Verification items for the finished model (mm, model axes). A direction names the side the tool comes from. Round coordinates to 2 decimals unless told otherwise and drop trailing zeros. Write each loop counter-clockwise with the first axis right and the second up, starting at its lowest first coordinate (ties: lowest second). Pieces come first, ordered by that corner, then holes. Notation, with made-up numbers: M 65,-28.75 L 101,-28.75 A18 cw 101,-8.75 Z; hole C -15,28 d4. An arc over 180 degrees is marked long. Answer in a Markdown table with one row per item. Add a question column.
1. Go/stop test with flat-tipped pins: pin 1 Ø2 at (y, z) = (4, 0) entering from +X; pin 2 Ø1.2 at (y, z) = (-3.5, 0.5) entering from -X; pin 3 Ø4 at (x, y) = (-127, 0) entering from +Z; pin 4 Ø2 at (x, z) = (93, 1) entering from -Y. Record where each tip stops, or that it passes through.
2. Draft check along X on faces 1 (the flat face through (2, 0, 2)), 2 (the cylindrical face through (135, 0, 0)), 3 (the cylindrical face through (-110.3, 9.57, 0.03)). Enter one of: pulls with the +X half, pulls with the -X half, needs draft (parallel to the pull), parting line crosses it, or undercut.
3. Sectioned sample at B-B on z = -0.5. Count the separate pieces of the cut face and the enclosed holes in it, plus the area to 3 significant figures.
4. Material ranges on probe 1 along Y at (x, z) = (28.5, 0.2); probe 2 along X at (y, z) = (-12, -1.2); probe 3 along Y at (x, z) = (110.5, -0.1), recorded low to high.
5. Set-up check for faces 4 (the cylindrical face through (-135, 0, 0)), 5 (the cylindrical face through (101, -9, 0)): record each of +Z, -Z, +X, -X, +Y, -Y from which the full face is reachable in a straight line by a thin tool's end or side.
6. Sectioned sample at A-A on x = -127. Record the cut outline in (y, z), plus the area to 3 significant figures.
```python
from build123d import *

# Parameters (mm, degrees)
EXTRUDE_1_DEPTH     = 2
SKETCH_11_W         = 4.2
SKETCH_11_H         = 15
SKETCH_11_W_2       = 46.8
SKETCH_11_H_2       = 22
SKETCH_11_W_3       = 5
SKETCH_11_R         = 3.5
SKETCH_11_R_2       = 1.5
CUT_EXTRUDE_1_DEPTH = 10
SKETCH_12_W         = 45
SKETCH_12_H         = 22
EXTRUDE_2_DEPTH     = 4
SKETCH_13_W         = 4.1
SKETCH_13_H         = 15
CUT_EXTRUDE_2_DEPTH = 136.889661123
FILLET_1_R          = 5


with BuildPart() as part:
    # Эскиз1 → Бобышка-Вытянуть1 (new, symmetric)
    with BuildSketch(Plane.XY):
        with BuildLine():
            Line((-120, 15), (120, 15))
            ThreePointArc((120, 15), (135, 0), (120, -15))
            Line((120, -15), (-120, -15))
            ThreePointArc((-120, -15), (-135, 0), (-120, 15))
        make_face()
    extrude(amount=EXTRUDE_1_DEPTH, both=True)

    # Эскиз11 → Вырез-Вытянуть1 (cut)
    with BuildSketch(Plane(origin=(0, 0, -2), x_dir=(-1, 0, 0), z_dir=(0, 0, -1))):
        with Locations((-117.9, 7.5)):
            Rectangle(SKETCH_11_W, SKETCH_11_H)
        with Locations((-88.4, 0)):
            Rectangle(SKETCH_11_W_2, SKETCH_11_H_2)
        with Locations((-57.5, 0)):
            Rectangle(SKETCH_11_W_3, SKETCH_11_H_2)
        with Locations((-47.5, 0)):
            Rectangle(SKETCH_11_W_3, SKETCH_11_H_2)
        with Locations((-37.5, 0)):
            Rectangle(SKETCH_11_W_3, SKETCH_11_H_2)
        with Locations((-27.5, 0)):
            Rectangle(SKETCH_11_W_3, SKETCH_11_H_2)
        with Locations((-17.5, 0)):
            Rectangle(SKETCH_11_W_3, SKETCH_11_H_2)
        with Locations((-7.5, 0)):
            Rectangle(SKETCH_11_W_3, SKETCH_11_H_2)
        with Locations((7.5, 0)):
            Rectangle(SKETCH_11_W_3, SKETCH_11_H_2)
        with Locations((17.5, 0)):
            Rectangle(SKETCH_11_W_3, SKETCH_11_H_2)
        with Locations((27.5, 0)):
            Rectangle(SKETCH_11_W_3, SKETCH_11_H_2)
        with Locations((37.5, 0)):
            Rectangle(SKETCH_11_W_3, SKETCH_11_H_2)
        with Locations((47.5, 0)):
            Rectangle(SKETCH_11_W_3, SKETCH_11_H_2)
        with Locations((57.5, 0)):
            Rectangle(SKETCH_11_W_3, SKETCH_11_H_2)
        with Locations((88.4, 0)):
            Rectangle(SKETCH_11_W_2, SKETCH_11_H_2)
        with Locations((117.9, 7.5)):
            Rectangle(SKETCH_11_W, SKETCH_11_H)
        with Locations((127, 0)):
            Circle(SKETCH_11_R)
        with Locations((-127, 0)):
            Circle(SKETCH_11_R)
        Circle(SKETCH_11_R_2)
        with Locations((-120, -8)):
            Circle(SKETCH_11_R_2)
        with Locations((120, -8)):
            Circle(SKETCH_11_R_2)
    extrude(amount=-CUT_EXTRUDE_1_DEPTH, mode=Mode.SUBTRACT)

    # Эскиз12 → Бобышка-Вытянуть2 (add)
    with BuildSketch(Plane.XY.offset(2)):
        with Locations((-77.5, 0)):
            Rectangle(SKETCH_12_W, SKETCH_12_H)
    extrude_2 = extrude(amount=-EXTRUDE_2_DEPTH)

    # Зеркальное отражение1: Бобышка-Вытянуть2 across plane
    add(extrude_2.mirror(Plane(origin=(0, 0, 0), x_dir=(0, 0, 1), z_dir=(1, 0, 0))))

    # Эскиз13 → Вырез-Вытянуть2 (cut, through all)
    with BuildSketch(Plane.XY.offset(2)):
        with Locations((-92.05, -7.5)):
            Rectangle(SKETCH_13_W, SKETCH_13_H)
    cut_extrude_2 = extrude(amount=-CUT_EXTRUDE_2_DEPTH, mode=Mode.SUBTRACT)

    # Зеркальное отражение2: Вырез-Вытянуть2 across plane
    add(cut_extrude_2.mirror(Plane(origin=(0, 0, 0), x_dir=(0, 0, 1), z_dir=(1, 0, 0))), mode=Mode.SUBTRACT)

    # Скругление1
    fillet_1_edges = [part.edges().sort_by_distance(p)[0] for p in [
        (-111.8, 11, 0),
        (-111.8, -11, 0),
        (-100, 11, 0),
        (-100, -11, 0),
        (100, -11, 0),
        (100, 11, 0),
        (111.8, -11, 0),
        (111.8, 11, 0),
    ]]
    fillet(fillet_1_edges, radius=FILLET_1_R)


solid = part.part
```
Geometry check:
| question | item | result |
|---|---|---|
| 1 | pin 1 | stops at x = 134.7 |
| 1 | pin 2 | stops at x = -134.72 |
| 1 | pin 3 | passes through |
| 1 | pin 4 | stops at y = 0 |
| 2 | face 1 | needs draft |
| 2 | face 2 | pulls with the +X half |
| 2 | face 3 | undercut |
| 3 | separate pieces | 1 |
| 3 | enclosed holes | 17 |
| 3 | area | 5,980 mm2 |
| 4 | probe 1 | y = -15 to -11, 11 to 15 |
| 4 | probe 2 | x = -129 to -94.1, -90 to 90, 94.1 to 129 |
| 4 | probe 3 | y = -15 to -9.36, 9.36 to 15 |
| 5 | face 4 | +Z, -Z, -X |
| 5 | face 5 | +Z, -Z |
| 6 | outline | M -13.27,-2 L -3.5,-2 L -3.5,2 L -13.27,2 Z; M 3.5,-2 L 13.27,-2 L 13.27,2 L 3.5,2 Z |
| 6 | area | 78.1 mm2 |
